Could you check a few things on this drawing? It's one solid part, dimensions in mm from its lowest x, y, z. A direction names the side the tool comes from. Round coordinates to 2 decimals unless told otherwise and drop trailing zeros. Write each loop counter-clockwise with the first axis right and the second up, starting at its lowest first coordinate (ties: lowest second). Pieces come first, ordered by that corner, then holes. Notation, with made-up numbers: (-17.5, -32.5) -> (20.5, -32.5) arc R10 ccw to (20.5, -20.5) -> close; hole circle Ø3 at (52, -3.75). An arc over 180 degrees is marked (long way). Return JSON: item names as keys, results as strings.
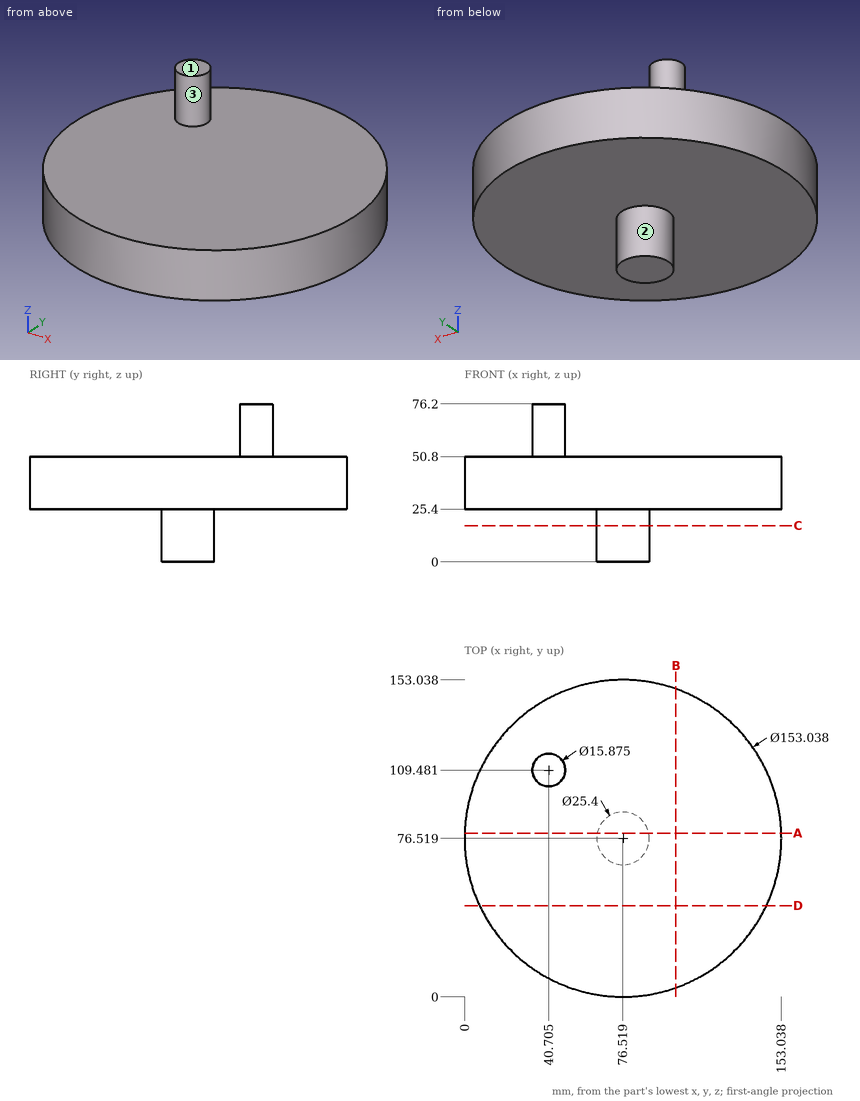
1) For the marked faces 1, 2 and 3, which set-ups out of +Z, -Z, +X, -X, +Y, -Y let a thin tool reach every point of the face, with its end or its side?
Return value:
{"face 1": "+Z, +X, -X, +Y, -Y", "face 2": "-Z", "face 3": "+Z"}
2) If I drill on probe 1 along Z at (x, y) = (7, 80.5); probe 2 along Z at (x, y) = (80.5, 70); probe 3 along Y at (x, z) = (76, 31.5), over which ranges is the centre line in solid material (lowest first)? Write a range as [from, to].
Return value:
{"probe 1": "[25.4, 50.8]", "probe 2": "[0, 50.8]", "probe 3": "[0, 153.04]"}
3) I want a section at C-C, the plane z = 17.5. Please give me the cut outline in (x, y).
Return value:
{"outline": "circle Ø25.4 at (76.52, 76.52)"}
4) I want a section at B-B, the plane x = 102. Please give me the cut outline in (y, z), and give its area (3 significant figures).
Return value:
{"outline": "(4.37, 25.4) -> (148.67, 25.4) -> (148.67, 50.8) -> (4.37, 50.8) -> close", "area": "3,670 mm²"}
5) I want a section at A-A, the plane y = 79. Please give me the cut outline in (x, z) (1 decimal), and give its area (3 significant figures).
Return value:
{"outline": "(0, 25.4) -> (64.1, 25.4) -> (64.1, 0) -> (89, 0) -> (89, 25.4) -> (153, 25.4) -> (153, 50.8) -> (0, 50.8) -> close", "area": "4,520 mm²"}
6) I want a section at D-D, the plane y = 44. Please give me the cut outline in (x, z) (1 decimal).
Return value:
{"outline": "(7.3, 25.4) -> (145.8, 25.4) -> (145.8, 50.8) -> (7.3, 50.8) -> close"}
7) Will these pins go through, and if not, where does the flat tip stop? pin 1 Ø2 at (y, z) = (42, 47) entering from -X; pin 2 Ø3 at (y, z) = (105, 64) entering from +X; pin 3 Ø12 at (x, y) = (16, 66.5) entering from -Z.
Return value:
{"pin 1": "x = 7.73", "pin 2": "x = 48.06", "pin 3": "z = 25.4"}
